```python
from build123d import *

# Parameters (mm, degrees)
SKETCH1_W               = 44
SKETCH1_H               = 44
BOSS_EXTRUDE1_DEPTH     = 5
SKETCH2_W               = 36
SKETCH2_H               = 36
BOSS_EXTRUDE2_DEPTH     = 1.8
CUT_EXTRUDE1_REACH      = 51.447
SKETCH3_W               = 5
SKETCH3_H               = 3.2
SKETCH4_W               = 44
SKETCH4_H               = 44
SKETCH4_W_2             = 30
SKETCH4_H_2             = 30
BOSS_EXTRUDE3_DEPTH     = 2
FILLET1_R               = 1
TAP_DRILL_FOR_M3_TAP1_D = 2.5


with BuildPart() as part:
    # Sketch1 → Boss-Extrude1 (new body)
    with BuildSketch(Plane(origin=(0, 0, 0), x_dir=(1, 0, 0), z_dir=(0, 1, 0))):
        Rectangle(SKETCH1_W, SKETCH1_H)
        Polygon((20.1, -20.1), (20.1, 21.1), (18.1, 21.1), (18.1, 20.1), (-18.1, 20.1), (-18.1, 21.1), (-20.1, 21.1), (-20.1, -20.1), align=None, mode=Mode.SUBTRACT)
    extrude(amount=BOSS_EXTRUDE1_DEPTH)

    # Sketch2 → Boss-Extrude2 (add)
    with BuildSketch(Plane(origin=(0, 5, 0), x_dir=(1, 0, 0), z_dir=(0, 1, 0))):
        Polygon((-20.1, 21.1), (-20.1, -20.1), (20.1, -20.1), (20.1, 21.1), (18.1, 21.1), (18.1, 20.1), (-18.1, 20.1), (-18.1, 21.1), align=None)
        Rectangle(SKETCH2_W, SKETCH2_H, mode=Mode.SUBTRACT)
    extrude(amount=-BOSS_EXTRUDE2_DEPTH)

    # Sketch3 → Cut-Extrude1 (cut, up to next)
    with BuildSketch(Plane.XY.offset(22), mode=Mode.PRIVATE) as cut_extrude1_sk1:
        with Locations((-17.6, 1.6)):
            Rectangle(SKETCH3_W, SKETCH3_H)
    cut_extrude1_tool1 = extrude(cut_extrude1_sk1.sketch, amount=-CUT_EXTRUDE1_REACH, mode=Mode.PRIVATE) & part.part
    # Sketch3 → Cut-Extrude1 (cut, up to next)
    with BuildSketch(Plane.XY.offset(22), mode=Mode.PRIVATE) as cut_extrude1_sk2:
        with Locations((17.6, 1.6)):
            Rectangle(SKETCH3_W, SKETCH3_H)
    cut_extrude1_tool2 = extrude(cut_extrude1_sk2.sketch, amount=-CUT_EXTRUDE1_REACH, mode=Mode.PRIVATE) & part.part
    add(cut_extrude1_tool1.solids().sort_by_distance((-17.6, 1.6, 22))[0], mode=Mode.SUBTRACT)
    add(cut_extrude1_tool2.solids().sort_by_distance((17.6, 1.6, 22))[0], mode=Mode.SUBTRACT)

    # Sketch4 → Boss-Extrude3 (add)
    with BuildSketch(Plane(origin=(0, 5, 0), x_dir=(1, 0, 0), z_dir=(0, 1, 0))):
        Rectangle(SKETCH4_W, SKETCH4_H)
        Rectangle(SKETCH4_W_2, SKETCH4_H_2, mode=Mode.SUBTRACT)
    extrude(amount=BOSS_EXTRUDE3_DEPTH)

    # Fillet1
    fillet1_edges = [part.edges().sort_by_distance(p)[0] for p in [
        (-18, 4.1, 18),
        (18, 4.1, 18),
        (18, 4.1, -18),
        (-18, 4.1, -18),
        (-20.1, 1.6, -21.1),
        (-18.1, 1.6, -21.1),
        (18.1, 1.6, -21.1),
        (20.1, 1.6, -21.1),
        (-15, 6, -15),
        (-15, 6, 15),
        (15, 6, -15),
        (15, 6, 15),
    ]]
    fillet(fillet1_edges, radius=FILLET1_R - 0.0001)  # a hair under: the kernel refuses the full size

    # Tap Drill for M3 Tap1 (through all)
    with Locations(Plane(origin=(0, 7, 0), x_dir=(1, 0, 0), z_dir=(0, 1, 0))):
        with Locations((-16, 16), (16, 16), (16, -16), (-16, -16)):
            Hole(TAP_DRILL_FOR_M3_TAP1_D / 2)


solid = part.part
```
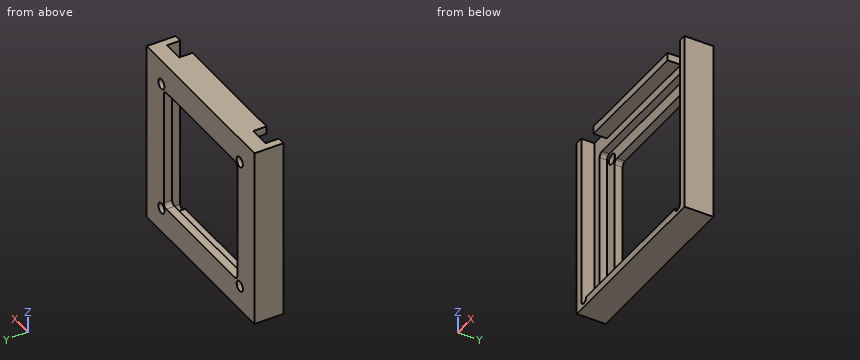
Can you work these out from the model? Positions are in its coordinate system, mm. Give positions to 0.01 mm unless a question says otherwise; leave off trailing zeros. Loops run counter-clockwise (first coordinate to the right, second up) from the corner with the lowest first, then second, coordinate; pieces in that order, holes last. Notation, with made-up numbers: M 18.5,65 L 70.5,65 A16 cw 70.5,83 Z; hole C 12.25,-20 d10. An arc over 180 degrees is marked long. Use CSV: the item, a comma, the result in double quotes. Start each with the question number.
1. For P1, Ø12, axis at x = 6.5, z = -9.5, coming from the -Y side, with a flat end and sliding along its axis, tell me the tip position at first contact or that it passes through.
2. Imagine slicing it at A-A, the plane z = -7. Write out the boundary of the cut face in (x, y).
3. Imagine slicing it at C-C, the plane x = 7.5. Write out the boundary of the cut face in (y, z), plus the area to 3 significant figures.
4. If I drill on L1, parallel to Z at x = 16, y = 6.1; L2, parallel to Z at x = 5.5, y = 3.5, over which ranges is the centre line in solid material (lowest first)?
5. Imagine slicing it at D-D, the plane z = 16. Write out the boundary of the cut face in (x, y), plus the area to 3 significant figures.
Response values:
1,P1,"y = 5"
2,outline,"M -22,0 L -20.1,0 L -20.1,3.2 L -18,3.2 L -18,5 L -15,5 L -15,7 L -22,7 Z; M 15,5 L 18,5 L 18,3.2 L 20.1,3.2 L 20.1,0 L 22,0 L 22,7 L 15,7 Z"
3,outline,"M 0,-22 L 7,-22 L 7,-15 L 5,-15 L 5,-18 L 3.2,-18 L 3.2,-20.1 L 0,-20.1 Z; M 0,20.1 L 3.2,20.1 L 3.2,18 L 5,18 L 5,15 L 7,15 L 7,22 L 0,22 Z"
3,area,"54.6 mm^2"
4,L1,"-22 to -17.25, -14.75 to 14.75, 17.25 to 22"
4,L2,"-22 to -18, 18 to 22"
5,outline,"M -22,0 L -20.1,0 L -20.1,3.2 L -18,3.2 L -18,5 L -17.25,5 L -17.25,7 L -22,7 Z; M -14.75,5 L 14.75,5 L 14.75,7 L -14.75,7 Z; M 17.25,5 L 18,5 L 18,3.2 L 20.1,3.2 L 20.1,0 L 22,0 L 22,7 L 17.25,7 Z"
5,area,"105 mm^2"
